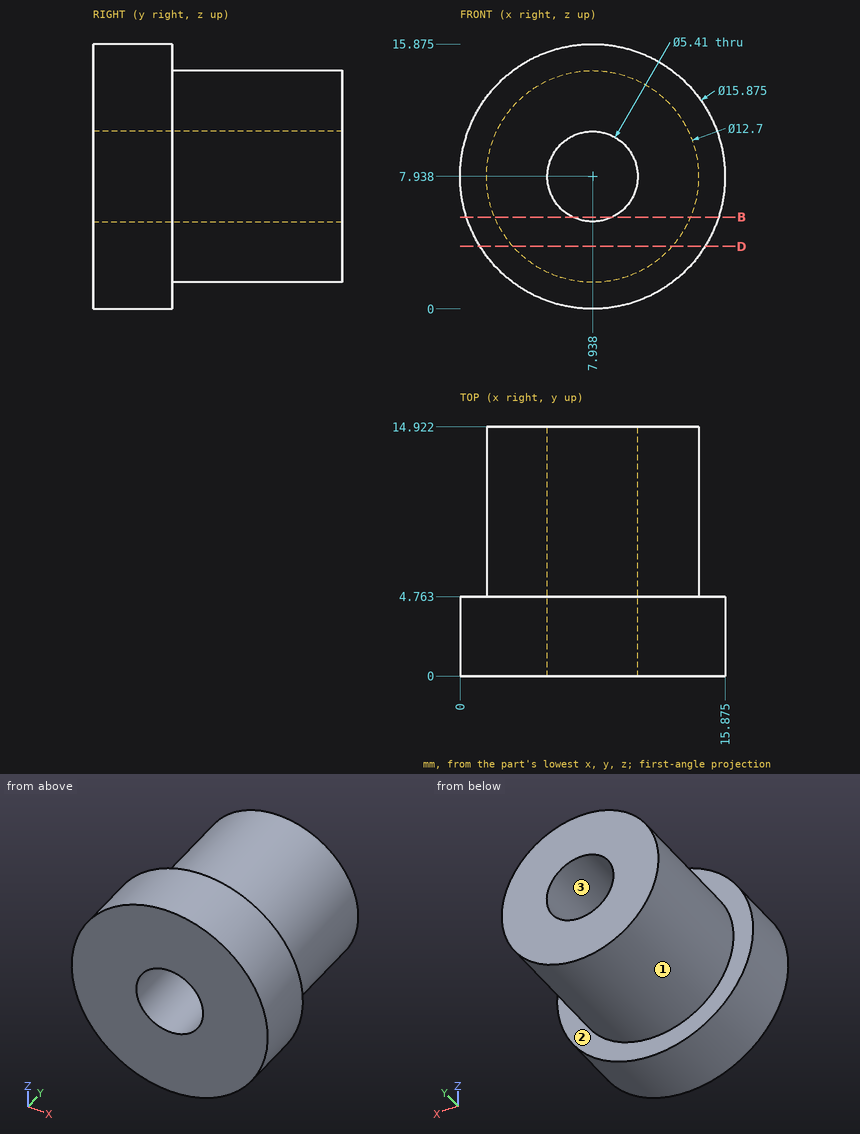
Geometry check sheet. Reference: drawing and pictorial views, mm from the part's lowest x, y, z. Round coordinates to 2 decimals unless told otherwise and drop trailing zeros. Loops run counter-clockwise (first coordinate to the right, second up) from the corner with the lowest first, then second, coordinate; pieces in that order, holes last.
1. Mould release check, pull along Z, two halves, no side actions. Record for the marked faces 1, 2 and 3: released by +Z, released by -Z, zero draft, split by the parting line, or undercut.
2. Sectioned sample at B-B on z = 5.5. Record the boundary of the cut face in (x, y) (1 decimal), and give its area (3 significant figures).
3. Scan lines: probe 1 along X at (y, z) = (5.75, 8); probe 2 along Y at (x, z) = (6, 15.25); probe 3 along Z at (x, y) = (9.5, 7.75) (1 decimal). Record each from-to range of solid material in increasing order.
4. Gauge pin test, flat ends, axial feed: pin 1 Ø1.5 at (x, z) = (14, 2) entering from +Y; pin 2 Ø1 at (y, z) = (3, 4.5) entering from -X; pin 3 Ø5 at (x, y) = (11.5, 8.5) entering from -Z. Record the tip position at first contact, or that the pin passes through.
5. Sectioned sample at D-D on z = 3.75. Record the boundary of the cut face in (x, y) (1 decimal).
Recorded:
1. face 1: split by the parting line
1. face 2: zero draft
1. face 3: undercut
2. outline: (0.4, 0) - (6.8, 0) - (6.8, 14.9) - (2.1, 14.9) - (2.1, 4.8) - (0.4, 4.8) - close; (9.1, 0) - (15.5, 0) - (15.5, 4.8) - (13.8, 4.8) - (13.8, 14.9) - (9.1, 14.9) - close
2. area: 156 mm2
3. probe 1: x = 1.59 to 5.23, 10.64 to 14.29
3. probe 2: y = 0 to 4.76
3. probe 3: z = 1.8 to 5.7, 10.1 to 14.1
4. pin 1: stops at y = 4.76
4. pin 2: stops at x = 0.56
4. pin 3: stops at z = 1.68
5. outline: (1.2, 0) - (14.7, 0) - (14.7, 4.8) - (12.7, 4.8) - (12.7, 14.9) - (3.2, 14.9) - (3.2, 4.8) - (1.2, 4.8) - close
